Read the model definition and answer for the solid it produces. Units are mm, in the model's axes. A direction names the side the tool comes from. Give positions to 0.01 mm unless a question says otherwise; leave off trailing zeros. Write each loop counter-clockwise with the first axis right and the second up, starting at its lowest first coordinate (ties: lowest second). Pieces come first, ordered by that corner, then holes. Notation, with made-up numbers: M 37.5,25.5 L 68.5,25.5 A15 ccw 68.5,45.5 Z; hole C -15,39.25 d4. An arc over 180 degrees is marked long. Put each result on its own line as item: value.
from build123d import *

# Parameters (mm, degrees)
F0_W      = 63.5
F0_H      = 150
F1_DEPTH  = 1.5
F2_W      = 47.5
F2_H      = 39.9
F2_H_2    = 38.8
F2_H_3    = 39.3
F3_DEPTH  = 1.501
F4_R      = 8
F5_W      = 63.5
F5_H      = 0.5
F6_DEPTH  = 4
F7_W      = 5
F7_H      = 0.8
F8_DEPTH  = 5.25
F9_W      = 5
F9_H      = 0.8
F10_DEPTH = 5.25
F11_W     = 4.5
F11_H     = 0.6
F12_DEPTH = 5
F13_W     = 4.5
F13_H     = 0.6
F14_DEPTH = 5
F15_W     = 2.25
F15_H     = 5
F16_DEPTH = 5.501
F17_W     = 2
F17_H     = 4.5
F18_DEPTH = 0.9
F19_W     = 2
F19_H     = 4.5
F20_DEPTH = 0.9
F21_W     = 2
F21_H     = 4.5
F22_DEPTH = 0.9
F23_W     = 2
F23_H     = 4.5
F24_DEPTH = 0.9
F25_W     = 2
F25_H     = 4.5
F26_DEPTH = 0.9
F27_W     = 2
F27_H     = 4.5
F28_DEPTH = 0.9
F29_SIZE  = 1


with BuildPart() as f1:
    # F0 (on Top) → F1 (new body)
    with BuildSketch(Plane.XY):
        with Locations((31.75, 75)):
            Rectangle(F0_W, F0_H)
    extrude(amount=F1_DEPTH)

    # F2 (on face) → F3 (cut, through all)
    with BuildSketch(Plane.XY.offset(1.5)):
        with Locations((31.75, 122.05)):
            Rectangle(F2_W, F2_H)
        with Locations((31.75, 74.7)):
            Rectangle(F2_W, F2_H_2)
        with Locations((31.75, 27.65)):
            Rectangle(F2_W, F2_H_3)
    extrude(amount=-F3_DEPTH, mode=Mode.SUBTRACT)

    # F4
    f4_edges = [f1.edges().sort_by_distance(p)[0] for p in [
        (8, 142, 0.75),
        (8, 94.1, 0.75),
        (8, 47.3, 0.75),
        (8, 102.1, 0.75),
        (8, 55.3, 0.75),
        (8, 8, 0.75),
        (55.5, 102.1, 0.75),
        (55.5, 55.3, 0.75),
        (55.5, 8, 0.75),
        (55.5, 142, 0.75),
        (55.5, 94.1, 0.75),
        (55.5, 47.3, 0.75),
    ]]
    fillet(f4_edges, radius=F4_R)

    # F5 (on face) → F6 (join)
    with BuildSketch(Plane.XY.offset(1.5)):
        with Locations((31.75, 0.25)):
            Rectangle(F5_W, F5_H)
        with Locations((31.75, 149.75)):
            Rectangle(F5_W, F5_H)
    extrude(amount=F6_DEPTH)

    # F7 (on face) → F8 (cut)
    with BuildSketch(Plane.YZ.offset(63.5)):
        with Locations((142.5, 1.1)):
            Rectangle(F7_W, F7_H)
        with Locations((77.5, 1.1)):
            Rectangle(F7_W, F7_H)
        with Locations((12.5, 1.1)):
            Rectangle(F7_W, F7_H)
    extrude(amount=-F8_DEPTH, mode=Mode.SUBTRACT)

    # F9 (on face) → F10 (cut)
    with BuildSketch(Plane(origin=(0, 0, 0), x_dir=(0, -1, 0), z_dir=(-1, 0, 0))):
        with Locations((-7.5, 1.1)):
            Rectangle(F9_W, F9_H)
        with Locations((-72.5, 1.1)):
            Rectangle(F9_W, F9_H)
        with Locations((-137.5, 1.1)):
            Rectangle(F9_W, F9_H)
    extrude(amount=-F10_DEPTH, mode=Mode.SUBTRACT)

    # F11 (on face) → F12 (join)
    with BuildSketch(Plane(origin=(0, 0, 0), x_dir=(0, -1, 0), z_dir=(-1, 0, 0))):
        with Locations((-142.5, 1.2)):
            Rectangle(F11_W, F11_H)
        with Locations((-77.5, 1.2)):
            Rectangle(F11_W, F11_H)
        with Locations((-12.5, 1.2)):
            Rectangle(F11_W, F11_H)
    extrude(amount=F12_DEPTH)

    # F13 (on face) → F14 (join)
    with BuildSketch(Plane.YZ.offset(63.5)):
        with Locations((137.5, 1.2)):
            Rectangle(F13_W, F13_H)
        with Locations((72.5, 1.2)):
            Rectangle(F13_W, F13_H)
        with Locations((7.5, 1.2)):
            Rectangle(F13_W, F13_H)
    extrude(amount=F14_DEPTH)

    # F15 (on face) → F16 (cut, through all)
    with BuildSketch(Plane(origin=(0, 0, 0), x_dir=(1, 0, 0), z_dir=(0, 0, -1))):
        with Locations((59.375, -12.5)):
            Rectangle(F15_W, F15_H)
        with Locations((4.125, -7.5)):
            Rectangle(F15_W, F15_H)
        with Locations((59.375, -77.5)):
            Rectangle(F15_W, F15_H)
        with Locations((4.125, -72.5)):
            Rectangle(F15_W, F15_H)
        with Locations((59.375, -142.5)):
            Rectangle(F15_W, F15_H)
        with Locations((4.125, -137.5)):
            Rectangle(F15_W, F15_H)
    extrude(amount=-F16_DEPTH, mode=Mode.SUBTRACT)

    # F17 (on face) → F18 (join)
    with BuildSketch(Plane(origin=(0, 0, 0.9), x_dir=(1, 0, 0), z_dir=(0, 0, -1))):
        with Locations((-4, -12.5)):
            Rectangle(F17_W, F17_H)
    extrude(amount=F18_DEPTH)

    # F19 (on face) → F20 (join)
    with BuildSketch(Plane(origin=(0, 0, 0.9), x_dir=(1, 0, 0), z_dir=(0, 0, -1))):
        with Locations((-4, -77.5)):
            Rectangle(F19_W, F19_H)
    extrude(amount=F20_DEPTH)

    # F21 (on face) → F22 (join)
    with BuildSketch(Plane(origin=(0, 0, 0.9), x_dir=(1, 0, 0), z_dir=(0, 0, -1))):
        with Locations((-4, -142.5)):
            Rectangle(F21_W, F21_H)
    extrude(amount=F22_DEPTH)

    # F23 (on face) → F24 (join)
    with BuildSketch(Plane(origin=(0, 0, 0.9), x_dir=(1, 0, 0), z_dir=(0, 0, -1))):
        with Locations((67.5, -137.5)):
            Rectangle(F23_W, F23_H)
    extrude(amount=F24_DEPTH)

    # F25 (on face) → F26 (join)
    with BuildSketch(Plane(origin=(0, 0, 0.9), x_dir=(1, 0, 0), z_dir=(0, 0, -1))):
        with Locations((67.5, -72.5)):
            Rectangle(F25_W, F25_H)
    extrude(amount=F26_DEPTH)

    # F27 (on face) → F28 (join)
    with BuildSketch(Plane(origin=(0, 0, 0.9), x_dir=(1, 0, 0), z_dir=(0, 0, -1))):
        with Locations((67.5, -7.5)):
            Rectangle(F27_W, F27_H)
    extrude(amount=F28_DEPTH)

    # F29
    f29_edges = [f1.edges().sort_by_distance(p)[0] for p in [
        (-5, 142.5, 0),
        (-5, 77.5, 0),
        (-5, 12.5, 0),
        (68.5, 72.5, 0),
        (68.5, 137.5, 0),
        (68.5, 7.5, 0),
    ]]
    chamfer(f29_edges, length=F29_SIZE)


solid = f1.part
(1) Section D-D on y = 137.5 is taken. Determine the outline of the cut face in (x, z).
Result:
outline: M 0,0 L 3,0 L 3,0.7 L 0,0.7 Z; M 5.25,0 L 8.81,0 L 8.81,1.5 L 5.25,1.5 Z; M 54.69,0 L 63.5,0 L 63.5,0.9 L 66.5,0.9 L 66.5,0 L 67.5,0 L 68.5,1 L 68.5,1.5 L 54.69,1.5 Z
(2) For a pull along Y with two mould halves and no side action, classify faces 6 (the face through (65, 7, 0.9)), 7 (the face through (31, 0, 3)), 8 (the face through (1, 8, 0.7)) as +Y half, -Y half, draft (parallel to the pull), parting line (faces both ways), or undercut.
Result:
face 6: draft
face 7: -Y half
face 8: undercut
(3) Section A-A on x = 44.5 is taken. Determine the outline of the cut face in (y, z), and give its area (3 significant figures).
Result:
outline: M 0,0 L 8,0 L 8,1.5 L 0.5,1.5 L 0.5,5.5 L 0,5.5 Z; M 47.3,0 L 55.3,0 L 55.3,1.5 L 47.3,1.5 Z; M 94.1,0 L 102.1,0 L 102.1,1.5 L 94.1,1.5 Z; M 142,0 L 150,0 L 150,5.5 L 149.5,5.5 L 149.5,1.5 L 142,1.5 Z
area: 52.0 mm²
(4) Which of the six approach directions +Z, -Z, +X, -X, +Y, -Y give full straight-line access (tool end or side, diameter ignored) to faces 1 (the face through (62, 77, 0.7)), 2 (the face through (1, 138, 0.7)), 3 (the face through (-1, 78, 0.9)), 4 (the face through (31, 149.5, 3)), 5 (the face through (53.219, 44.894, 0.74))?
Result:
face 1: +Z, +X
face 2: +Z, -X
face 3: -Z, +Y, -Y
face 4: +Z, +X, -X
face 5: +Z, -Z
(5) Given pin 1 Ø1.5 at (x, y) = (2, 138) entering from +Z; pin 2 Ø1.2 at (y, z) = (12.5, 1) entering from +X; pin 3 Ø3 at (y, z) = (126.5, 4) entering from -X; pin 4 Ø1.6 at (y, z) = (123, 0.5) entering from -X, each flat-ended and moving along its own axis, determine where each tip first touches the part or whether it passes through.
Result:
pin 1: stops at z = 0.7
pin 2: stops at x = 63.5
pin 3: passes through
pin 4: stops at x = 0
(6) Straight lines are drawn through the part: line 1 along Y through (x, z) = (17, 2.5); line 2 along X through (y, z) = (129.5, 1); line 3 along Y through (x, z) = (50.5, 0.75). For each, find the intervals that lie inside material, in ascending order. Write a range as from..to.
Result:
line 1: y = 0..0.5, 149.5..150
line 2: x = 0..8, 55.5..63.5
line 3: y = 0..8.58, 46.72..55.88, 93.52..102.68, 141.42..150
(7) Section B-B on y = 36.5 is taken. Determine the outline of the cut face in (x, z).
Result:
outline: M 0,0 L 8,0 L 8,1.5 L 0,1.5 Z; M 55.5,0 L 63.5,0 L 63.5,1.5 L 55.5,1.5 Z
(8) Section C-C on z = 4.15 is taken. Determine the outline of the cut face in (x, y), and give its area (3 significant figures).
Result:
outline: M 0,0 L 63.5,0 L 63.5,0.5 L 0,0.5 Z; M 0,149.5 L 63.5,149.5 L 63.5,150 L 0,150 Z
area: 63.5 mm²
